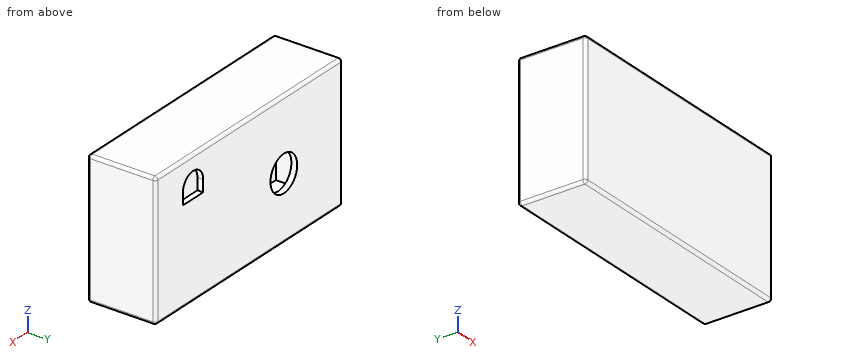
from build123d import *

# Parameters (mm, degrees)
SKETCH1_W           = 222.25
SKETCH1_H           = 59.69
BOSS_EXTRUDE1_DEPTH = 118.11
FILLET1_R           = 2.54
SHELL1_T            = 5.08
SKETCH2_R           = 15.875
CUT_EXTRUDE1_DEPTH  = 7.62


with BuildPart() as part:
    # Sketch1 → Boss-Extrude1 (new body)
    with BuildSketch(Plane.XY):
        with Locations((111.125, 29.845)):
            Rectangle(SKETCH1_W, SKETCH1_H)
    extrude(amount=BOSS_EXTRUDE1_DEPTH)

    # Fillet1
    fillet1_edges = [part.edges().sort_by_distance(p)[0] for p in [
        (222.25, 29.845, 118.11),
        (111.125, 59.69, 118.11),
        (0, 29.845, 118.11),
        (111.125, 59.69, 0),
        (222.25, 29.845, 0),
        (111.125, 0, 0),
        (0, 29.845, 0),
        (111.125, 0, 118.11),
        (0, 59.69, 59.055),
        (222.25, 59.69, 59.055),
        (222.25, 0, 59.055),
        (0, 0, 59.055),
    ]]
    fillet(fillet1_edges, radius=FILLET1_R)

    # Shell1 (no face opened: a closed hollow body)
    add(offset(amount=-SHELL1_T, mode=Mode.PRIVATE), mode=Mode.SUBTRACT)

    # Sketch2 → Cut-Extrude1 (cut)
    with BuildSketch(Plane(origin=(0, 59.69, 0), x_dir=(1, 0, 0), z_dir=(0, 1, 0))):
        with Locations(Location((69.85, -55.88, 0), (0, 0, 270))):  # turned: the seam where the file's is
            Circle(SKETCH2_R)
        with BuildLine():
            Line((165.735, -82.423), (189.865, -82.423))
            Line((189.865, -82.423), (189.865, -92.71))
            ThreePointArc((189.865, -92.71), (177.8, -104.775), (165.735, -92.71))
            Line((165.735, -92.71), (165.735, -82.423))
        make_face()
    extrude(amount=-CUT_EXTRUDE1_DEPTH, mode=Mode.SUBTRACT)


solid = part.part
Design review of the part built by this model. Coordinates are the model's own, in mm. Give positions to 0.01 mm unless a question says otherwise; leave off trailing zeros. Order: outer loops, then holes, each group sorted by start corner. A loop starts at its lowest first (then second) coordinate and runs counter-clockwise, first axis right, second up.
1. Add section D-D, the plane x = 177.8. State the section outline as (y, z) points (3 decimals).
Solution:
outline: (0, 2.54) arc R2.54 ccw to (2.54, 0) - (57.15, 0) arc R2.54 ccw to (59.69, 2.54) - (59.69, 82.423) - (54.61, 82.423) - (54.61, 5.08) - (5.08, 5.08) - (5.08, 113.03) - (54.61, 113.03) - (54.61, 104.775) - (59.69, 104.775) - (59.69, 115.57) arc R2.54 ccw to (57.15, 118.11) - (2.54, 118.11) arc R2.54 ccw to (0, 115.57) - close
2. Add section C-C, the plane z = 55.88. State the section outline as (x, y) points (3 decimals).
Solution:
outline: (0, 2.54) arc R2.54 ccw to (2.54, 0) - (219.71, 0) arc R2.54 ccw to (222.25, 2.54) - (222.25, 57.15) arc R2.54 ccw to (219.71, 59.69) - (85.725, 59.69) - (85.725, 54.61) - (217.17, 54.61) - (217.17, 5.08) - (5.08, 5.08) - (5.08, 54.61) - (53.975, 54.61) - (53.975, 59.69) - (2.54, 59.69) arc R2.54 ccw to (0, 57.15) - close
3. To check wall thickness, follow L1, parallel to Y at x = 58, z = 15; L2, parallel to X at y = 9, z = 95; L3, parallel to X at y = 57, z = 55. State the ranges of each line that lie inside material, in increasing order.
Solution:
L1: y = 0 to 5.08, 54.61 to 59.69
L2: x = 0 to 5.08, 217.17 to 222.25
L3: x = 0 to 54, 85.7 to 222.25
4. Add section A-A, the plane x = 143. State the section outline as (y, z) points.
Solution:
outline: (0, 2.54) arc R2.54 ccw to (2.54, 0) - (57.15, 0) arc R2.54 ccw to (59.69, 2.54) - (59.69, 115.57) arc R2.54 ccw to (57.15, 118.11) - (2.54, 118.11) arc R2.54 ccw to (0, 115.57) - close; hole (5.08, 5.08) - (54.61, 5.08) - (54.61, 113.03) - (5.08, 113.03) - close
5. Add section B-B, the plane y = 9. State the section outline as (x, z) points.
Solution:
outline: (0, 2.54) arc R2.54 ccw to (2.54, 0) - (219.71, 0) arc R2.54 ccw to (222.25, 2.54) - (222.25, 115.57) arc R2.54 ccw to (219.71, 118.11) - (2.54, 118.11) arc R2.54 ccw to (0, 115.57) - close; hole (5.08, 5.08) - (217.17, 5.08) - (217.17, 113.03) - (5.08, 113.03) - close
